Geometry check sheet. Reference: the model listing, model coordinates, mm. A direction names the side the tool comes from. Round coordinates to 2 decimals unless told otherwise and drop trailing zeros. Order: outer loops, then holes, each group sorted by start corner. A loop starts at its lowest first (then second) coordinate and runs counter-clockwise, first axis right, second up. Notation, with made-up numbers: (35.5, 5) - (46.5, 5) arc R18 cw to (46.5, 29) - close; hole circle Ø4 at (89.5, 88.25). An arc over 180 degrees is marked (long way). One line per question, with ' | ' between items. Start each with the question number.
Q1. Sectioned sample at A-A, the plane x = 1. Enter the section's corners in (y, z).
Q2. Mould release check, pull along X, two halves, no side actions. Record for faces 5 (the face through (1, 7.5, 9)), 6 (the face through (0, 0, 3.721)), 7 (the face through (-9.96, 0.2, 8.1)), 8 (the face through (0, -6, -4)): +X half, -X half, draft (parallel to the pull), parting line (faces both ways), or undercut.
Q3. Gauge pin test, flat ends, axial feed: P1, Ø1.5, axis at x = 14.5, y = 0, coming from the -Z side; P2, Ø2, axis at x = -7.5, z = 8, coming from the -Y side; P3, Ø1.6, axis at x = 1, y = 3.5, coming from the +Z side. Record the tip position at first contact, or that the pin passes through.
Q4. Sectioned sample at C-C, the plane z = 8. Give the number of separate pieces and of enclosed holes in the cut face, then the cut area to 3 significant figures.
Q5. Sectioned sample at D-D, the plane x = 5. Enter the section's corners in (y, z), then the cut area to 3 significant figures.
Q6. Sectioned sample at B-B, the plane x = -11. Enter the section's corners in (y, z), then the cut area to 3 significant figures.
Q7. Material ranges on line 1 along X through (y, z) = (-9, -8.25); line 2 along Z through (x, y) = (-3.5, -8.75); line 3 along Y through (x, z) = (-4, -12.25), recorded low to high.
Q8. Tool access check on faces 1 (the face through (-9, 0, 9.521)), 2 (the face through (-8, 5, 8)), 3 (the face through (-2.769, 5.206, -2.825)), 4 (the face through (0, -10.334, 1)). Record the directions out of +Z, -Z, +X, -X, +Y, -Y that give a thin tool (end or side, any length) a straight path to the whole face; none if there is none.
```python
from build123d import *

# Parameters (mm, degrees)
SKETCH3_R                = 14.933526733
BOSS_EXTRUDE2_DEPTH      = 5
SKETCH4_W                = 3.6
SKETCH4_H                = 15
CUT_EXTRUDE1_DEPTH       = 2
CUT_EXTRUDE1_DEPTH_BACK  = 30.620731291
CUT_EXTRUDE4_START       = 4
SKETCH6_W                = 5.202489895
SKETCH6_H                = 21.176797573
CUT_EXTRUDE4_DEPTH       = 34.154759474
SKETCH8_R                = 1
CUT_EXTRUDE6_DEPTH       = 5
SKETCH9_R                = 1
CUT_EXTRUDE9_DEPTH       = 5
SKETCH10_W               = 3.6
SKETCH10_H               = 15
BOSS_EXTRUDE3_DEPTH      = 15
CUT_EXTRUDE10_START      = -5
SKETCH11_W               = 0.8
SKETCH11_H               = 15
CUT_EXTRUDE10_DEPTH      = 12
SKETCH12_R               = 1.55
CUT_EXTRUDE11_DEPTH      = 30.154759474
CUT_EXTRUDE11_DEPTH_BACK = 30.154759474


with BuildPart() as part:
    # Sketch1 → Revolve2 (revolve)
    with BuildSketch(Plane.XY, mode=Mode.PRIVATE) as revolve2_sk:
        Polygon((0, 0), (0, 15), (20, 0), align=None)
    revolve(revolve2_sk.sketch.rotate(Axis((-31.294130364, 0, 0), (1, 0, 0)), 90), axis=Axis((-31.294130364, 0, 0), (1, 0, 0)))

    # Sketch3 → Boss-Extrude2 (add)
    with BuildSketch(Plane(origin=(0, 0, 0), x_dir=(0, 0, -1), z_dir=(1, 0, 0))):
        Circle(SKETCH3_R)
    extrude(amount=-BOSS_EXTRUDE2_DEPTH)

    # Sketch4 → Cut-Extrude1 (cut, two sides)
    with BuildSketch(Plane(origin=(0, 0, -0.886715275), x_dir=(0, 0, -1), z_dir=(1, 0, 0))) as cut_extrude1_sk:
        with Locations((-9.407876673, 0)):
            Rectangle(SKETCH4_W, SKETCH4_H)
    extrude(amount=CUT_EXTRUDE1_DEPTH, mode=Mode.SUBTRACT)
    extrude(cut_extrude1_sk.sketch, amount=-CUT_EXTRUDE1_DEPTH_BACK, mode=Mode.SUBTRACT)

    # Sketch6 → Cut-Extrude4 (cut, through all)
    with BuildSketch(Plane(origin=(0, 0, 0), x_dir=(0, 0, -1), z_dir=(1, 0, 0)).offset(CUT_EXTRUDE4_START)):
        with Locations((-1.119916451, 0.254630833)):
            Rectangle(SKETCH6_W, SKETCH6_H)
    extrude(amount=-CUT_EXTRUDE4_DEPTH, mode=Mode.SUBTRACT)

    # Sketch8 → Cut-Extrude6 (cut)
    with BuildSketch(Plane.XY):
        with Locations((-2.552019749, 6.182563449)):
            Circle(SKETCH8_R)
        with Locations(Location((-2.552019749, -6.182563449, 0), (0, 0, 270))):
            Circle(SKETCH8_R)
    extrude(amount=-CUT_EXTRUDE6_DEPTH, mode=Mode.SUBTRACT)

    # Sketch9 → Cut-Extrude9 (cut)
    with BuildSketch(Plane(origin=(0, 0, 0), x_dir=(0, 0, -1), z_dir=(1, 0, 0))):
        with Locations((3.923175217, -6.295020596)):
            Circle(SKETCH9_R)
        with Locations((3.923175217, 6.295020596)):
            Circle(SKETCH9_R)
    extrude(amount=-CUT_EXTRUDE9_DEPTH, mode=Mode.SUBTRACT)

    # Sketch10 → Boss-Extrude3 (add)
    with BuildSketch(Plane(origin=(0, 0, 0), x_dir=(0, 0, -1), z_dir=(1, 0, 0))):
        with Locations((-8.521161398, 0)):
            Rectangle(SKETCH10_W, SKETCH10_H)
    extrude(amount=-BOSS_EXTRUDE3_DEPTH)

    # Sketch11 → Cut-Extrude10 (cut)
    with BuildSketch(Plane(origin=(0, 0, 0), x_dir=(0, 0, -1), z_dir=(1, 0, 0)).offset(CUT_EXTRUDE10_START)):
        with Locations((-9.921161398, 0)):
            Rectangle(SKETCH11_W, SKETCH11_H)
    extrude(amount=-CUT_EXTRUDE10_DEPTH, mode=Mode.SUBTRACT)

    # Sketch12 → Cut-Extrude11 (cut, two sides)
    with BuildSketch(Plane.XY) as cut_extrude11_sk:
        with BuildLine():
            ThreePointArc((-15, 0), (-13.535533906, 3.535533906), (-10, 5))
            Line((-10, 5), (-5, 5))
            Line((-5, 5), (-5, 9.202194168))
            Line((-5, 9.202194168), (-18.010498555, 9.996270698))
            Line((-18.010498555, 9.996270698), (-16.284245229, -10.269943354))
            Line((-16.284245229, -10.269943354), (-5, -9.308764033))
            Line((-5, -9.308764033), (-5, -5))
            Line((-5, -5), (-10, -5))
            ThreePointArc((-10, -5), (-13.535533906, -3.535533906), (-15, 0))
        make_face()
        with Locations(Location((-11.495940447, 0, 0), (0, 0, 270))):
            Circle(SKETCH12_R)
    extrude(amount=CUT_EXTRUDE11_DEPTH, mode=Mode.SUBTRACT)
    extrude(cut_extrude11_sk.sketch, amount=-CUT_EXTRUDE11_DEPTH_BACK, mode=Mode.SUBTRACT)


solid = part.part
```
Determined:
1) outline: circle Ø28.5 at (0, 0); hole (-10.33, -1.48) - (10.84, -1.48) - (10.84, 3.72) - (-10.33, 3.72) - close; hole (-7.5, 6.72) - (7.5, 6.72) - (7.5, 10.32) - (-7.5, 10.32) - close
2) face 5: undercut | face 6: draft | face 7: undercut | face 8: -X half
3) P1: stops at z = -4.69 | P2: stops at y = -5 | P3: stops at z = 14.46
4) separate pieces: 1 | enclosed holes: 2 | area: 326 mm2
5) outline: circle Ø22.5 at (0, 0) | area: 398 mm2
6) outline: (-4.9, 6.72) - (-1.47, 6.72) - (-1.47, 9.52) - (-4.9, 9.52) - close; (1.47, 6.72) - (4.9, 6.72) - (4.9, 9.52) - (1.47, 9.52) - close | area: 19.2 mm2
7) line 1: x = -5 to 3.72 | line 2: z = -12.1 to -1.48, 3.72 to 12.1 | line 3: y = -8.54 to 8.54
8) face 1: +Z, -X, +Y, -Y | face 2: +Z, -Z, -X, +Y | face 3: none | face 4: -X
